from build123d import *

# Parameters (mm, degrees)
F0_W     = 50.8
F0_H     = 25.4
F1_DEPTH = 3.175
F2_W     = 1.5875
F2_H     = 3.81
F3_DEPTH = 25.4
F5_DEPTH = 3.175


with BuildPart() as f1:
    # F0 (on Top) → F1 (new body)
    with BuildSketch(Plane.XY):
        with Locations((25.4, -12.7)):
            Rectangle(F0_W, F0_H)
    extrude(amount=F1_DEPTH)

    # F2 (on face) → F3 (join)
    with BuildSketch(Plane.XY.offset(3.175)):
        with Locations((26.19375, -14.605)):
            Rectangle(F2_W, F2_H)
        with Locations((24.60625, -14.605)):
            Rectangle(F2_W, F2_H)
        with Locations((26.19375, -10.795)):
            Rectangle(F2_W, F2_H)
        with Locations((24.60625, -10.795)):
            Rectangle(F2_W, F2_H)
    extrude(amount=F3_DEPTH)

    # F4 (on face) → F5 (cut, through all)
    with BuildSketch(Plane.YZ.offset(26.9875)):
        Polygon((-14.9225, 15.875), (-16.51, 15.875), (-16.51, 8.255), align=None)
    extrude(amount=-F5_DEPTH, mode=Mode.SUBTRACT)


solid = f1.part
Could you check a few things on this model? Use its own coordinates, in mm. A direction names the side the tool comes from. Coordinates: 2 decimals unless noted, no trailing zeros. Order: outer loops, then holes, each group sorted by start corner. A loop starts at its lowest first (then second) coordinate and runs counter-clockwise, first axis right, second up.
Q1. Please list where these lines run through material, in increasing order: L1, parallel to Z at x = 24.5, y = -17.75 (3 decimals); L2, parallel to X at y = -11.5, z = 15.25; L3, parallel to Y at x = 25, z = 26.
Q2. Suppose I cut it at A-A on y = -11.5. Please give me the cut outline in (x, z) (1 decimal), and give its area (3 significant figures).
Q3. Will these pins go through, and if not, where does the flat tip stop? pin 1 (8.5 mm diameter, centred on y = -13, z = 15, fed in from -X); pin 2 (10 mm diameter, centred on y = -8.5, z = 23.5, fed in from +X); pin 3 (3.5 mm diameter, centred on x = 26, z = 24.5, fed in from -Y).
Q4. Suppose I cut it at C-C on x = 15. Please give me the cut outline in (y, z) (3 decimals), and give its area (3 significant figures).
Q5. Which directions (+Z, -Z, +X, -X, +Y, -Y) give clear straight access to the entire face, cutting with the end or side of a thin tool? Please do faces 1 (the flat face through (25, -8.89, 16)), 2 (the flat face through (26.988, -13, 16)), 3 (the flat face through (25, -16.51, 22)), 4 (the flat face through (23.812, -13, 16)), 5 (the flat face through (25, -16, 15.875)).
Q6. Suppose I cut it at D-D on z = 24.25. Please give me the cut outline in (x, y), and give its area (3 significant figures).
Q7. Suppose I cut it at B-B on y = -15.5. Please give me the cut outline in (x, z) (1 decimal), and give its area (3 significant figures).
Answer:
1. L1: z = 0 to 3.175
1. L2: x = 23.81 to 26.99
1. L3: y = -16.51 to -8.89
2. outline: (0, 0) - (50.8, 0) - (50.8, 3.2) - (27, 3.2) - (27, 28.6) - (23.8, 28.6) - (23.8, 3.2) - (0, 3.2) - close
2. area: 242 mm2
3. pin 1: stops at x = 23.81
3. pin 2: stops at x = 26.99
3. pin 3: stops at y = -16.51
4. outline: (-25.4, 0) - (0, 0) - (0, 3.175) - (-25.4, 3.175) - close
4. area: 80.6 mm2
5. face 1: +Z, +X, -X, +Y
5. face 2: +Z, +X, +Y, -Y
5. face 3: +Z, +X, -X, -Y
5. face 4: +Z, -X, +Y, -Y
5. face 5: +X, -X, -Y
6. outline: (23.81, -16.51) - (26.99, -16.51) - (26.99, -8.89) - (23.81, -8.89) - close
6. area: 24.2 mm2
7. outline: (0, 0) - (50.8, 0) - (50.8, 3.2) - (27, 3.2) - (27, 13.1) - (23.8, 13.1) - (23.8, 3.2) - (0, 3.2) - close; (23.8, 15.9) - (27, 15.9) - (27, 28.6) - (23.8, 28.6) - close
7. area: 233 mm2
